Work out the finished part from the listing and answer in its coordinate system (mm). A direction names the side the tool comes from. Round coordinates to 2 decimals unless told otherwise and drop trailing zeros. Loops run counter-clockwise (first coordinate to the right, second up) from the corner with the lowest first, then second, coordinate; pieces in that order, holes last. Notation, with made-up numbers: (62, 22) - (90, 22) arc R33 ccw to (90, 56) - close; hole circle Ø2 at (-3.75, -5.5). An arc over 180 degrees is marked (long way). Return JSON: item names as keys, results as strings.
from build123d import *

# Parameters (mm, degrees)
SWEEP1_PROFILE_R     = 6
SWEEP2_PROFILE_R     = 6
CUT_SWEEP1_PROFILE_R = 5
CUT_SWEEP2_PROFILE_R = 5


with BuildPart() as part:
    # Sweep1: sweep along a path in Sketch1
    with BuildLine(Plane(origin=(0, 0, 0), x_dir=(0, 0, -1), z_dir=(1, 0, 0))) as sweep1_path:
        Line((0, 5), (0, 0))
        ThreePointArc((0, 0), (-1.534261237, -7.271825561), (-5.87549411, -13.30399778))
        ThreePointArc((-5.87549411, -13.30399778), (-10.770150151, -20.105155205), (-12.5, -28.30399778))
        Line((-12.5, -28.30399778), (-12.5, -38.30399778))
    # Sweep1 profile (on start of the path) → Sweep1 (sweep)
    with BuildSketch(Plane(origin=(0, 5, 0), x_dir=(0, 0, -1), z_dir=(0, -1, 0))):
        Circle(SWEEP1_PROFILE_R)
    sweep(path=sweep1_path.line)

    # Sweep2: sweep along a path in Sketch3
    with BuildLine(Plane(origin=(0, 0, 0), x_dir=(0, 0, -1), z_dir=(1, 0, 0))) as sweep2_path:
        Line((12.5, -38.30399778), (12.5, -28.30399778))
        ThreePointArc((12.5, -28.30399778), (10.770150151, -20.105155205), (5.87549411, -13.30399778))
        ThreePointArc((5.87549411, -13.30399778), (1.534261237, -7.271825561), (0, 0))
        Line((0, 0), (0, 5))
    # Sweep2 profile (on start of the path) → Sweep2 (sweep)
    with BuildSketch(Plane(origin=(0, -38.30399778, -12.5), x_dir=(0, 0, 1), z_dir=(0, 1, 0))):
        Circle(SWEEP2_PROFILE_R)
    sweep(path=sweep2_path.line)

    # Cut-Sweep1: sweep along a path in Sketch1_5
    with BuildLine(Plane(origin=(0, 0, 0), x_dir=(0, 0, -1), z_dir=(1, 0, 0))) as cut_sweep1_path:
        Line((0, 5), (0, 0))
        ThreePointArc((0, 0), (-1.534261237, -7.271825561), (-5.87549411, -13.30399778))
        ThreePointArc((-5.87549411, -13.30399778), (-10.770150151, -20.105155205), (-12.5, -28.30399778))
        Line((-12.5, -28.30399778), (-12.5, -38.30399778))
    # Cut-Sweep1 profile (on start of the path) → Cut-Sweep1 (sweep, cut)
    with BuildSketch(Plane(origin=(0, 5, 0), x_dir=(0, 0, -1), z_dir=(0, -1, 0))):
        Circle(CUT_SWEEP1_PROFILE_R)
    sweep(path=cut_sweep1_path.line, mode=Mode.SUBTRACT)

    # Cut-Sweep2: sweep along a path in Sketch3_2
    with BuildLine(Plane(origin=(0, 0, 0), x_dir=(0, 0, -1), z_dir=(1, 0, 0))) as cut_sweep2_path:
        Line((12.5, -38.30399778), (12.5, -28.30399778))
        ThreePointArc((12.5, -28.30399778), (10.770150151, -20.105155205), (5.87549411, -13.30399778))
        ThreePointArc((5.87549411, -13.30399778), (1.534261237, -7.271825561), (0, 0))
        Line((0, 0), (0, 5))
    # Cut-Sweep2 profile (on start of the path) → Cut-Sweep2 (sweep, cut)
    with BuildSketch(Plane(origin=(0, -38.30399778, -12.5), x_dir=(0, 0, 1), z_dir=(0, 1, 0))):
        Circle(CUT_SWEEP2_PROFILE_R)
    sweep(path=cut_sweep2_path.line, mode=Mode.SUBTRACT)

    # Sketch111 → Revolve1 (revolve)
    with BuildSketch(Plane(origin=(0, 0, 0), x_dir=(0, 0, -1), z_dir=(1, 0, 0)), mode=Mode.PRIVATE) as revolve1_sk:
        Polygon((6.5, -33.30399778), (4.5, -35.30399778), (6.5, -35.30399778), align=None)
    revolve1 = revolve(revolve1_sk.sketch.rotate(Axis((0, -38.30399778, -12.5), (0, 1, 0)), 180), axis=Axis((0, -38.30399778, -12.5), (0, 1, 0)))

    # Mirror1: Revolve1 across plane
    add(revolve1.mirror(Plane.XY))


solid = part.part
1) Determine the mould class of faces 5 (the conical face through (5.43, -33.43, 15.33)), 6 (the cylindrical face through (1.802, -30.769, -6.777)), 7 (the cylindrical face through (1.802, -36.783, -6.777)), 8 (the flat face through (-6, -35.304, -14)) for opening direction Y: pulls with the +Y half, pulls with the -Y half, needs draft (parallel to the pull), parting line crosses it, or undercut.
Verdict:
{"face 5": "undercut", "face 6": "undercut", "face 7": "needs draft", "face 8": "pulls with the -Y half"}
2) Flat-ended cylindrical pins translate along their axes: pin 1 (3 mm diameter, centred on y = -29, z = 8, fed in from -X); pin 2 (8 mm diameter, centred on x = -2.5, z = 11, fed in from -Y); pin 3 (8 mm diameter, centred on y = -23, z = -12.5, fed in from +X); pin 4 (2 mm diameter, centred on x = 1, y = -31.5, fed in from -Z). Find the tip coordinate at first contact, or state that the pin passes through.
Verdict:
{"pin 1": "stops at x = -5.2", "pin 2": "stops at y = -38.3", "pin 3": "stops at x = 6", "pin 4": "stops at z = -18.5"}
3) Section A-A (y = -29.5) is taken. Give the vertices of the cut face in (x, z), and give its area (3 significant figures).
Verdict:
{"outline": "circle Ø12 at (0, -12.5); circle Ø12 at (0, 12.5); hole circle Ø10 at (0, -12.5); hole circle Ø10 at (0, 12.5)", "area": "69.1 mm2"}
4) Find the intervals of material crossed by L1, parallel to X at y = 2.6, z = 0; L2, parallel to X at y = -34.25, z = 12.5, in increasing order.
Verdict:
{"L1": "x = -6 to -5, 5 to 6", "L2": "x = -6.95 to -5, 5 to 6.95"}
5) Section B-B (z = 5.5) is taken. Count the separate pieces of the cut face and the enclosed holes in it, and give its area (3 significant figures).
Verdict:
{"separate pieces": "2", "enclosed holes": "1", "area": "105 mm2"}
6) A tool of negligible diameter and unlimited length cuts with its end or side. For faces 1 (the flat face through (4, 5, 4)), 2 (the cylindrical face through (1.802, -30.839, 6.777)), 3 (the cylindrical face through (0, 2, 6)), 4 (the cylindrical face through (1.5, -33.23, -7.73)), from which of +Z, -Z, +X, -X, +Y, -Y can it reach the whole face along a straight path? Write none if from no direction.
Verdict:
{"face 1": "+Z, -Z, +X, -X, +Y", "face 2": "none", "face 3": "+Y", "face 4": "-Y"}
